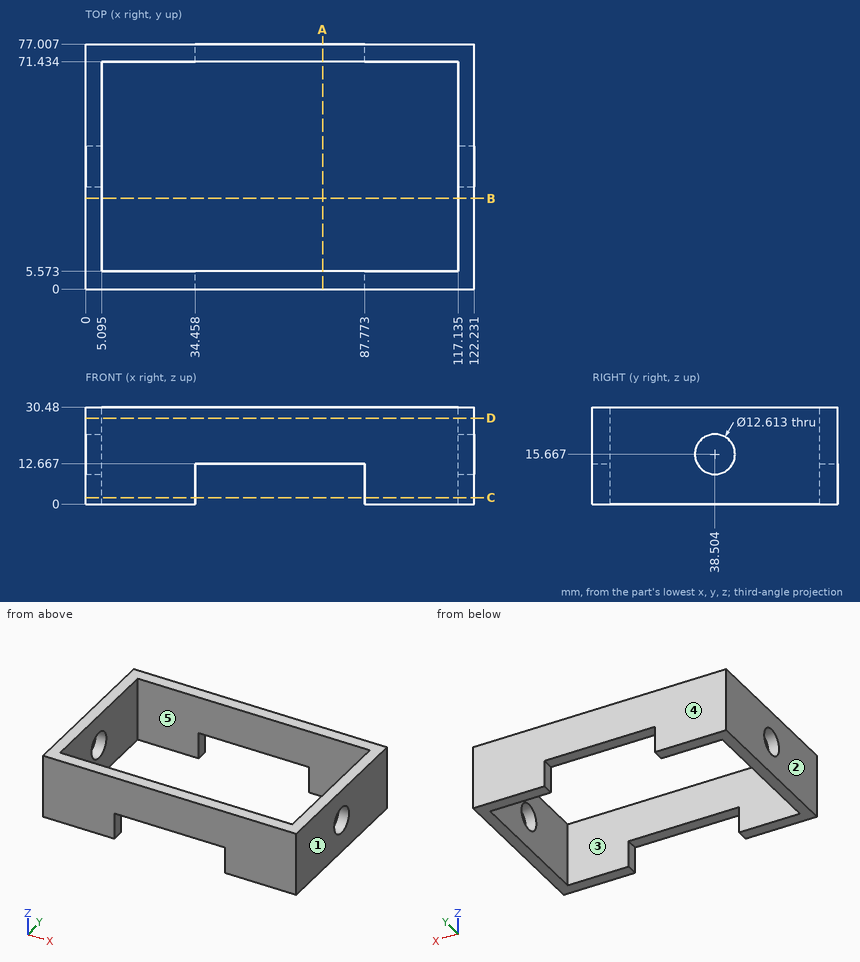
The drawing under review shows one solid part. Ordinate dimensions are in mm from its lowest x, y, z. A direction names the side the tool comes from. Round coordinates to 2 decimals unless told otherwise and drop trailing zeros. Loops run counter-clockwise (first coordinate to the right, second up) from the corner with the lowest first, then second, coordinate; pieces in that order, holes last.
Item 1: For the marked faces 4 and 5, list the 3-axis set-ups (+Z, -Z, +X, -X, +Y, -Y) from which the entire face can be reached by the end or side of a thin tool; tool diameter is ignored.
Determined:
face 4: +Z, -Z, +X, -X, +Y
face 5: +Z, -Z
Item 2: Take a section at A-A (x = 74.5). Write out the cut boundary in (y, z) (1 decimal).
Determined:
outline: (0, 12.7) - (5.6, 12.7) - (5.6, 30.5) - (0, 30.5) - close; (71.4, 12.7) - (77, 12.7) - (77, 30.5) - (71.4, 30.5) - close
Item 3: Mouldability with a two-part tool opening along X and no side actions: class the marked faces 1, 2 and 3 as released by +X, released by -X, zero draft, split by the parting line, or undercut.
Determined:
face 1: released by +X
face 2: released by -X
face 3: undercut
Item 4: Take a section at C-C (z = 2). Write out the cut boundary in (x, y) (1 decimal).
Determined:
outline: (0, 0) - (34.5, 0) - (34.5, 5.6) - (5.1, 5.6) - (5.1, 71.4) - (34.5, 71.4) - (34.5, 77) - (0, 77) - close; (87.8, 0) - (122.2, 0) - (122.2, 77) - (87.8, 77) - (87.8, 71.4) - (117.1, 71.4) - (117.1, 5.6) - (87.8, 5.6) - close
Item 5: Take a section at D-D (z = 27). Write out the cut boundary in (x, y) (1 decimal), then the cut area to 3 significant figures.
Determined:
outline: (0, 0) - (122.2, 0) - (122.2, 77) - (0, 77) - close; hole (5.1, 5.6) - (117.1, 5.6) - (117.1, 71.4) - (5.1, 71.4) - close
area: 2,030 mm2
Item 6: Take a section at B-B (y = 28.5). Write out the cut boundary in (x, z) (1 decimal).
Determined:
outline: (0, 0) - (5.1, 0) - (5.1, 30.5) - (0, 30.5) - close; (117.1, 0) - (122.2, 0) - (122.2, 30.5) - (117.1, 30.5) - close
Item 7: For line 1 (X direction, y = 63.5, z = 19) (1 decimal); line 2 (Y direction, x = 21, z = 16.5) (1 decimal), list the stretches that pass through material, from the lowest coordinate up.
Determined:
line 1: x = 0 to 5.1, 117.1 to 122.2
line 2: y = 0 to 5.6, 71.4 to 77
Item 8: Clearance check with a flat-ended pin moving along its axis: pin 1 Ø4.5 at (x, y) = (51, 75) entering from -Z. State where the tip first meets the part, or that it passes through.
Determined:
pin 1: stops at z = 12.67
